```python
from build123d import *

# Parameters (mm, degrees)
F0_W     = 25.4
F0_H     = 20.32
F1_DEPTH = 0.508
F2_W     = 25.3
F2_H     = 20.22
F3_DEPTH = 9.652
F4_R     = 0.5
F5_DEPTH = 0.1
F6_R     = 1
F7_R     = 0.254
F8_DEPTH = 3.81
F9_R     = 0.254


with BuildPart() as f1:
    # F0 (on Top) → F1 (new body)
    with BuildSketch(Plane.XY):
        with Locations((12.7, 10.16)):
            Rectangle(F0_W, F0_H)
    extrude(amount=F1_DEPTH)

    # F2 (on face) → F3 (join)
    with BuildSketch(Plane.XY.offset(0.508)):
        with Locations((12.7, 10.16)):
            Rectangle(F2_W, F2_H)
    extrude(amount=F3_DEPTH)

    # F4 (on face) → F5 (cut)
    with BuildSketch(Plane.XY.offset(10.16)):
        with Locations((3, 3)):
            Circle(F4_R)
    extrude(amount=-F5_DEPTH, mode=Mode.SUBTRACT)

    # F6
    f6_edges = [f1.edges().sort_by_distance(p)[0] for p in [
        (25.35, 0.05, 5.334),
        (25.35, 20.27, 5.334),
        (0.05, 0.05, 5.334),
        (0.05, 20.27, 5.334),
        (25.4, 0, 0.254),
        (25.4, 20.32, 0.254),
        (0, 0, 0.254),
        (0, 20.32, 0.254),
        (0.05, 10.16, 10.16),
        (12.7, 20.27, 10.16),
        (25.35, 10.16, 10.16),
        (12.7, 0.05, 10.16),
    ]]
    fillet(f6_edges, radius=F6_R)

    # F7 (on Top) → F8 (join)
    with BuildSketch(Plane.XY):
        with Locations((1.27, 2.794)):
            Circle(F7_R)
        with Locations((3.81, 2.794)):
            Circle(F7_R)
        with Locations((1.27, 18.034)):
            Circle(F7_R)
        with Locations((3.81, 18.034)):
            Circle(F7_R)
        with Locations((19.05, 18.034)):
            Circle(F7_R)
        with Locations((24.13, 18.034)):
            Circle(F7_R)
        with Locations((19.05, 2.794)):
            Circle(F7_R)
        with Locations((24.13, 2.794)):
            Circle(F7_R)
    extrude(amount=-F8_DEPTH)

    # F9
    f9_edges = [f1.edges().sort_by_distance(p)[0] for p in [
        (1.016, 2.794, -3.81),
        (3.556, 2.794, -3.81),
        (23.876, 2.794, -3.81),
        (18.796, 2.794, -3.81),
        (23.876, 18.034, -3.81),
        (18.796, 18.034, -3.81),
        (3.556, 18.034, -3.81),
        (1.016, 18.034, -3.81),
    ]]
    fillet(f9_edges, radius=F9_R)


solid = f1.part
```
Build history of the part. All positions in model axes, mm. A direction names the side the tool comes from. Coordinates: 2 decimals unless noted, no trailing zeros. Order: outer loops, then holes, each group sorted by start corner. A loop starts at its lowest first (then second) coordinate and runs counter-clockwise, first axis right, second up.
Item 1: Saw through at A-A on y = 16.75. List the corners of the cut face in (x, z), then the cut area to 3 significant figures.
Filled in:
outline: (0, 0) - (25.4, 0) - (25.4, 0.51) - (25.35, 0.51) - (25.35, 9.16) arc R1 ccw to (24.35, 10.16) - (1.05, 10.16) arc R1 ccw to (0.05, 9.16) - (0.05, 0.51) - (0, 0.51) - close
area: 257 mm2
Item 2: Mould opens along X. For faces 5 (the cylindrical face through (12.863, 0.335, 9.859)), 6 (the flat face through (25.35, 10, 5)), 7 (the flat face through (3, 3, 10.06)), 8 (the cylindrical face through (0.351, 0.335, 4.895)) say: released by +X, released by -X, zero draft, split by the parting line, or undercut.
Filled in:
face 5: zero draft
face 6: released by +X
face 7: undercut
face 8: released by -X
Item 3: Drill centre lines: L1, parallel to Z at x = 15.25, y = 8.25; L2, parallel to Y at x = 22.25, z = 1.25; L3, parallel to X at y = 19.25, z = 3.5. Where is each one in solid material? Low to high.
Filled in:
L1: z = 0 to 10.16
L2: y = 0.05 to 20.27
L3: x = 0.05 to 25.35
Item 4: Tool access for faces 1 (the flat face through (13, 20.27, 5)), 2 (the cylindrical face through (25.065, 19.969, 4.895)), 3 (the cylindrical face through (0.351, 19.985, 4.895)), 4 (the cylindrical face through (25.049, 0.335, 4.895)): list every direction of +Z, -Z, +X, -X, +Y, -Y with a clear straight run to the whole face (end or side of a thin tool).
Filled in:
face 1: +Z, +X, -X, +Y
face 2: +Z, +X, +Y
face 3: +Z, -X, +Y
face 4: +Z, +X, -Y
Item 5: Saw through at C-C on z = -0.5. List the corners of the cut face in (x, y).
Filled in:
outline: circle Ø0.51 at (1.27, 2.79); circle Ø0.51 at (1.27, 18.03); circle Ø0.51 at (3.81, 2.79); circle Ø0.51 at (3.81, 18.03); circle Ø0.51 at (19.05, 2.79); circle Ø0.51 at (19.05, 18.03); circle Ø0.51 at (24.13, 2.79); circle Ø0.51 at (24.13, 18.03)
Item 6: Drop flat-ended pins along their axis: pin 1 Ø3 at (y, z) = (10, 6.5) entering from +X; pin 2 Ø2.5 at (y, z) = (8.5, 5.5) entering from -X; pin 3 Ø3 at (x, z) = (9, 7) entering from -Y. Give the stop position or say it passes through.
Filled in:
pin 1: stops at x = 25.35
pin 2: stops at x = 0.05
pin 3: stops at y = 0.05
Item 7: Saw through at B-B on x = 7.5. List the corners of the cut face in (y, z), then the cut area to 3 significant figures.
Filled in:
outline: (0, 0) - (20.32, 0) - (20.32, 0.51) - (20.27, 0.51) - (20.27, 9.16) arc R1 ccw to (19.27, 10.16) - (1.05, 10.16) arc R1 ccw to (0.05, 9.16) - (0.05, 0.51) - (0, 0.51) - close
area: 205 mm2
Item 8: Saw through at D-D on x = 3. List the corners of the cut face in (y, z), then the cut area to 3 significant figures.
Filled in:
outline: (0, 0) - (20.32, 0) - (20.32, 0.51) - (20.27, 0.51) - (20.27, 9.16) arc R1 ccw to (19.27, 10.16) - (3.5, 10.16) - (3.5, 10.06) - (2.5, 10.06) - (2.5, 10.16) - (1.05, 10.16) arc R1 ccw to (0.05, 9.16) - (0.05, 0.51) - (0, 0.51) - close
area: 205 mm2
